from build123d import *

# Parameters (mm, degrees)
SKETCH1_W               = 70
SKETCH1_H               = 35
BOSS_EXTRUDE1_DEPTH     = 3
BOSS_EXTRUDE2_START     = -3
SKETCH3_W               = 35
SKETCH3_H               = 35
BOSS_EXTRUDE2_DEPTH     = 4
CUT_EXTRUDE1_DEPTH      = 40.752358421
CUT_EXTRUDE1_DEPTH_BACK = 40.752358421
SKETCH2_R               = 1.65
SKETCH2_R_2             = 11.25
SKETCH5_R               = 3
CUT_EXTRUDE3_DEPTH      = 2
SKETCH6_R               = 1.65
SKETCH6_W               = 16
SKETCH6_H               = 9
CUT_EXTRUDE4_DEPTH      = 40.33509883
SKETCH7_W               = 24
SKETCH7_H               = 24
CUT_EXTRUDE5_DEPTH      = 1.5
SKETCH8_W               = 7.5
SKETCH8_H               = 10
BOSS_EXTRUDE3_DEPTH     = 7
SKETCH9_W               = 10
SKETCH9_H               = 3
BOSS_EXTRUDE4_DEPTH     = 21
CUT_EXTRUDE6_REACH      = 43.56
SKETCH10_R              = 3


with BuildPart() as part:
    # Sketch1 → Boss-Extrude1 (new body)
    with BuildSketch(Plane(origin=(0, 0, 0), x_dir=(1, 0, 0), z_dir=(0, 1, 0))):
        Rectangle(SKETCH1_W, SKETCH1_H)
    extrude(amount=BOSS_EXTRUDE1_DEPTH)

    # Sketch3 → Boss-Extrude2 (add)
    with BuildSketch(Plane(origin=(0, 3, 0), x_dir=(1, 0, 0), z_dir=(0, 1, 0)).offset(BOSS_EXTRUDE2_START)):
        with Locations((-17.5, 0)):
            Rectangle(SKETCH3_W, SKETCH3_H)
    extrude(amount=-BOSS_EXTRUDE2_DEPTH)

    # Sketch2 → Cut-Extrude1 (cut, two sides: drawn at the far end of the back side and taken through both)
    with BuildSketch(Plane(origin=(0, 3, 0), x_dir=(1, 0, 0), z_dir=(0, 1, 0)).offset(-CUT_EXTRUDE1_DEPTH_BACK)):
        with Locations(Location((-30.5, 13, 0), (0, 0, 270))):
            Circle(SKETCH2_R)
        with Locations(Location((-4.5, 13, 0), (0, 0, 90))):
            Circle(SKETCH2_R)
        with Locations(Location((-4.5, -13, 0), (0, 0, 270))):
            Circle(SKETCH2_R)
        with Locations(Location((-30.5, -13, 0), (0, 0, 90))):
            Circle(SKETCH2_R)
        with Locations(Location((-17.5, 0, 0), (0, 0, 270))):
            Circle(SKETCH2_R_2)
    extrude(amount=CUT_EXTRUDE1_DEPTH + CUT_EXTRUDE1_DEPTH_BACK, mode=Mode.SUBTRACT)

    # Sketch5 → Cut-Extrude3 (cut)
    with BuildSketch(Plane(origin=(0, 3, 0), x_dir=(1, 0, 0), z_dir=(0, 1, 0))):
        with Locations(Location((-30.5, 13, 0), (0, 0, 270))):
            Circle(SKETCH5_R)
        with Locations(Location((-4.5, 13, 0), (0, 0, 90))):
            Circle(SKETCH5_R)
        with Locations(Location((-4.5, -13, 0), (0, 0, 270))):
            Circle(SKETCH5_R)
        with Locations(Location((-30.5, -13, 0), (0, 0, 90))):
            Circle(SKETCH5_R)
    extrude(amount=-CUT_EXTRUDE3_DEPTH, mode=Mode.SUBTRACT)

    # Sketch6 → Cut-Extrude4 (cut, through all)
    with BuildSketch(Plane.XZ):
        with Locations(Location((3.5, 8, 0), (0, 0, 270))):
            Circle(SKETCH6_R)
        with Locations(Location((19.5, 8, 0), (0, 0, 90))):
            Circle(SKETCH6_R)
        with Locations(Location((19.5, -8, 0), (0, 0, 270))):
            Circle(SKETCH6_R)
        with Locations(Location((3.5, -8, 0), (0, 0, 90))):
            Circle(SKETCH6_R)
        with Locations((11.5, 0)):
            Rectangle(SKETCH6_W, SKETCH6_H)
    extrude(amount=-CUT_EXTRUDE4_DEPTH, mode=Mode.SUBTRACT)

    # Sketch7 → Cut-Extrude5 (cut)
    with BuildSketch(Plane(origin=(0, 0, 0), x_dir=(-1, 0, 0), z_dir=(0, -1, 0))):
        with Locations((-12, 0)):
            Rectangle(SKETCH7_W, SKETCH7_H)
    extrude(amount=-CUT_EXTRUDE5_DEPTH, mode=Mode.SUBTRACT)

    # Sketch8 → Boss-Extrude3 (add)
    with BuildSketch(Plane(origin=(0, 3, 0), x_dir=(1, 0, 0), z_dir=(0, 1, 0))):
        with Locations((31.25, 0)):
            Rectangle(SKETCH8_W, SKETCH8_H)
    extrude(amount=BOSS_EXTRUDE3_DEPTH)

    # Sketch9 → Boss-Extrude4 (add)
    with BuildSketch(Plane.ZY.offset(-27.5)):
        with Locations((0, 8.5)):
            Rectangle(SKETCH9_W, SKETCH9_H)
    extrude(amount=BOSS_EXTRUDE4_DEPTH)

    # Sketch10 → Cut-Extrude6 (cut, up to next)
    with BuildSketch(Plane(origin=(0, 10, 0), x_dir=(1, 0, 0), z_dir=(0, 1, 0)), mode=Mode.PRIVATE) as cut_extrude6_sk1:
        with Locations(Location((11.5, 0, 0), (0, 0, 270))):
            Circle(SKETCH10_R)
    cut_extrude6_tool1 = extrude(cut_extrude6_sk1.sketch, amount=-CUT_EXTRUDE6_REACH, mode=Mode.PRIVATE) & part.part
    add(cut_extrude6_tool1.solids().sort_by_distance((11.5, 10, 0))[0], mode=Mode.SUBTRACT)


solid = part.part
The listing builds one solid part. Answer for the finished solid, in the listing's coordinates (mm). A direction names the side the tool comes from. Give positions to 0.01 mm unless a question says otherwise; leave off trailing zeros. Order: outer loops, then holes, each group sorted by start corner. A loop starts at its lowest first (then second) coordinate and runs counter-clockwise, first axis right, second up. Notation, with made-up numbers: (-15.75, 79) -> (-2.75, 79) arc R18 ccw to (-2.75, 94) -> close; hole circle Ø10 at (10, -21.5). An arc over 180 degrees is marked (long way). Put each result on its own line as item: value.
Item 1: A cutting plane is placed at C-C on x = -4.5. Give the vertices of the cut face in (y, z), plus the area to 3 significant figures.
Established:
outline: (-4, -17.5) -> (3, -17.5) -> (3, -16) -> (1, -16) -> (1, -14.65) -> (-4, -14.65) -> close; (-4, -11.35) -> (1, -11.35) -> (1, -10) -> (3, -10) -> (3, 10) -> (1, 10) -> (1, 11.35) -> (-4, 11.35) -> close; (-4, 14.65) -> (1, 14.65) -> (1, 16) -> (3, 16) -> (3, 17.5) -> (-4, 17.5) -> close
area: 188 mm^2
Item 2: A cutting plane is placed at B-B on z = -13. Give the vertices of the cut face in (x, y), plus the area to 3 significant figures.
Established:
outline: (-35, -4) -> (-32.15, -4) -> (-32.15, 1) -> (-33.5, 1) -> (-33.5, 3) -> (-35, 3) -> close; (-28.85, -4) -> (-6.15, -4) -> (-6.15, 1) -> (-7.5, 1) -> (-7.5, 3) -> (-27.5, 3) -> (-27.5, 1) -> (-28.85, 1) -> close; (-2.85, -4) -> (0, -4) -> (0, 0) -> (35, 0) -> (35, 3) -> (-1.5, 3) -> (-1.5, 1) -> (-2.85, 1) -> close
area: 293 mm^2
Item 3: Given P1, Ø3.5, axis at x = 21.5, y = 5.5, coming from the +Z side; P2, Ø5.5, axis at x = 18.5, y = 7.5, coming from the -Z side; P3, Ø1.6, axis at y = -2, z = 1, coming from the +X side, each flat-ended and moving along its own axis, determine where each tip first touches the part or whether it passes through.
Established:
P1: stops at z = 5
P2: stops at z = -5
P3: stops at x = 0
Item 4: For faces 4 (the face through (17, 7, 0)), 5 (the face through (-32, 1, -12)), 6 (the face through (24, 8, -5)), determine the directions among +Z, -Z, +X, -X, +Y, -Y from which every point of the face is accessible in a straight line to the end or side of a thin tool.
Established:
face 4: +Z, -Z, -X
face 5: +Y
face 6: -Z, +X, -X, +Y
Item 5: A cutting plane is placed at A-A on x = 26. Give the vertices of the cut face in (y, z), plus the area to 3 significant figures.
Established:
outline: (0, -17.5) -> (3, -17.5) -> (3, 17.5) -> (0, 17.5) -> close; (7, -5) -> (10, -5) -> (10, 5) -> (7, 5) -> close
area: 135 mm^2
Item 6: For a pull along X with two mould halves and no side action, classify faces 1 (the face through (-35, 0, 0)), 2 (the face through (3.57, 2.24, 9.65)), 3 (the face through (21, 10, 0)) as released by +X, released by -X, zero draft, split by the parting line, or undercut.
Established:
face 1: released by -X
face 2: undercut
face 3: zero draft
Item 7: A cutting plane is placed at D-D on y = -1. Give the vertices of the cut face in (x, z), plus the area to 3 significant figures.
Established:
outline: (-35, -17.5) -> (0, -17.5) -> (0, 17.5) -> (-35, 17.5) -> close; hole circle Ø3.3 at (-30.5, -13); hole circle Ø3.3 at (-30.5, 13); hole circle Ø22.5 at (-17.5, 0); hole circle Ø3.3 at (-4.5, -13); hole circle Ø3.3 at (-4.5, 13)
area: 793 mm^2
Item 8: Straight lines are drawn through the part: line 1 (X direction, y = -0.4, z = 13); line 2 (X direction, y = 1, z = 0); line 3 (Y direction, x = 21.5, z = 3.5). For each, find the intervals that lie inside material, in ascending order.
Established:
line 1: x = -35 to -32.15, -28.85 to -6.15, -2.85 to 0
line 2: x = -35 to -28.75, -6.25 to 0, 24 to 35
line 3: y = 1.5 to 3, 7 to 10
